Could you check a few things on this drawing? It's one solid part, dimensions in mm from its lowest x, y, z. A direction names the side the tool comes from. Give positions to 0.01 mm unless a question says otherwise; leave off trailing zeros. Loops run counter-clockwise (first coordinate to the right, second up) from the corner with the lowest first, then second, coordinate; pieces in that order, holes last. Notation, with made-up numbers: M -9,57 L 7,57 A30 cw 7,95 Z; hole C 89.25,29 d10. An arc over 180 degrees is marked long. Answer as a JSON object with one key per item and string values.
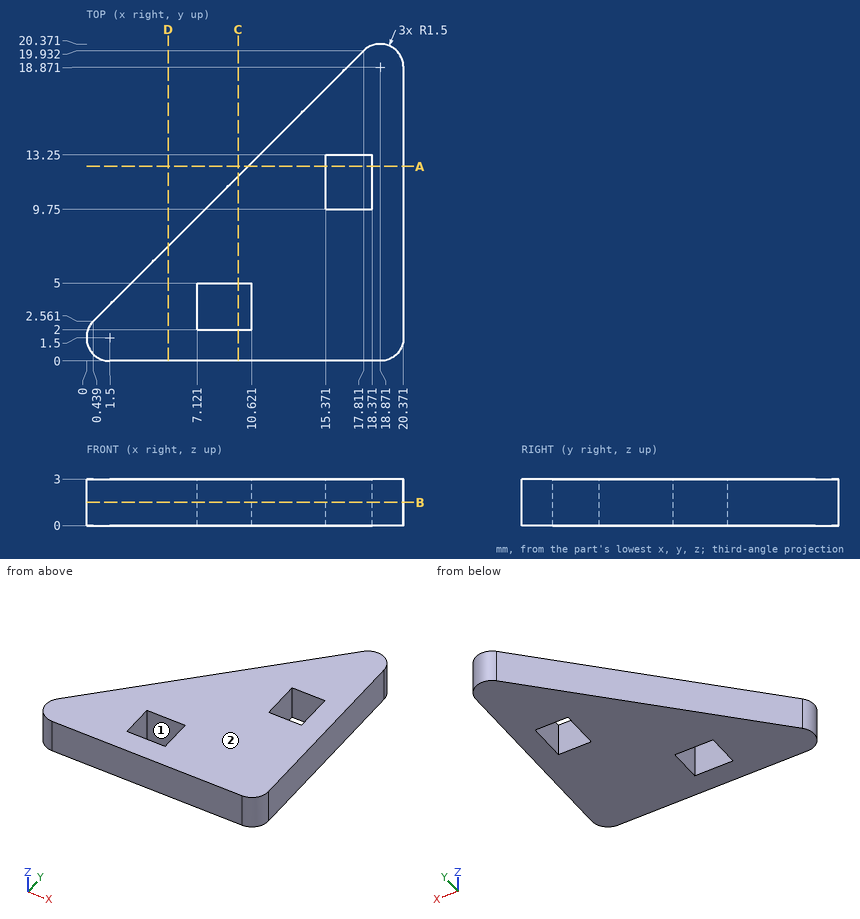
1) Will these pins go through, and if not, where does the flat tip stop? pin 1 Ø6 at (x, y) = (3.5, 10) entering from -Z; pin 2 Ø1.5 at (x, z) = (8.5, 2) entering from +Y.
Answer list:
{"pin 1": "through", "pin 2": "y = 11.37"}
2) Suppose I cut it at B-B, the plane z = 1.5. Write out the boundary of the cut face in (x, y).
Answer list:
{"outline": "M 0.44,2.56 A1.5 ccw 1.5,0 L 18.87,0 A1.5 ccw 20.37,1.5 L 20.37,18.87 A1.5 ccw 17.81,19.93 Z; hole M 7.12,2 L 10.62,2 L 10.62,5 L 7.12,5 Z; hole M 15.37,9.75 L 18.37,9.75 L 18.37,13.25 L 15.37,13.25 Z"}
3) For the marked faces 1 and 2, which set-ups out of +Z, -Z, +X, -X, +Y, -Y let a thin tool reach every point of the face, with its end or its side?
Answer list:
{"face 1": "+Z, -Z", "face 2": "+Z, +X, -X, +Y, -Y"}
4) Suppose I cut it at A-A, the plane y = 12.5. Write out the boundary of the cut face in (x, z).
Answer list:
{"outline": "M 10.38,0 L 15.37,0 L 15.37,3 L 10.38,3 Z; M 18.37,0 L 20.37,0 L 20.37,3 L 18.37,3 Z"}
5) Please list where these lines run through material, in increasing order: line 1 along Y through (x, z) = (9.5, 0.4); line 2 along Y through (x, z) = (9, 1.7); line 3 along X through (y, z) = (12.25, 1.2). Write a range as from..to.
Answer list:
{"line 1": "0..2, 5..11.62", "line 2": "0..2, 5..11.12", "line 3": "10.13..15.37, 18.37..20.37"}
6) Suppose I cut it at D-D, the plane x = 5.25. Write out the boundary of the cut face in (y, z), and give its area (3 significant figures).
Answer list:
{"outline": "M 0,0 L 7.37,0 L 7.37,3 L 0,3 Z", "area": "22.1 mm^2"}
7) Suppose I cut it at C-C, the plane x = 9.75. Write out the boundary of the cut face in (y, z), and give its area (3 significant figures).
Answer list:
{"outline": "M 0,0 L 2,0 L 2,3 L 0,3 Z; M 5,0 L 11.87,0 L 11.87,3 L 5,3 Z", "area": "26.6 mm^2"}
